Verification items for the finished model (mm, model axes). Face numbers are marked on the shaded views. A direction names the side the tool comes from. Round coordinates to 2 decimals unless told otherwise and drop trailing zeros. Write each loop counter-clockwise with the first axis right and the second up, starting at its lowest first coordinate (ties: lowest second). Pieces come first, ordered by that corner, then holes. Notation, with made-up numbers: (71.5, -23.75) - (82.5, -23.75) arc R26 cw to (82.5, -0.75) - close; hole circle Ø1 at (45.5, 78.25). An arc over 180 degrees is marked (long way). Write each question's results on one line, items separated by ' | '.
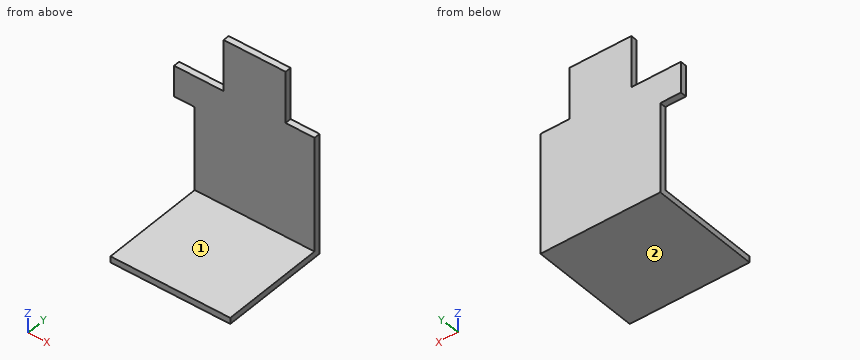
```python
from build123d import *

# Parameters (mm, degrees)
BOX015001038_W     = 58
BOX015001038_H     = 53.5
BOX015001038_DEPTH = 3
BOX015001039_W     = 10
BOX015001039_H     = 3
BOX015001039_DEPTH = 15
BOX015001041_W     = 14
BOX015001041_H     = 10
BOX015001041_DEPTH = 25
BOX015001040_W     = 14
BOX015001040_H     = 10
BOX015001040_DEPTH = 25
BOX015001037_W     = 58
BOX015001037_H     = 3
BOX015001037_DEPTH = 80.5


with BuildPart() as cube034:
    # Box015001038 → Box015001038 (new body)
    with BuildSketch(Plane(origin=(0, -50.5, -3), x_dir=(1, 0, 0), z_dir=(0, 0, 1))):
        with Locations((29, 26.75)):
            Rectangle(BOX015001038_W, BOX015001038_H)
    extrude(amount=BOX015001038_DEPTH)


with BuildPart() as cube035:
    # Box015001039 → Box015001039 (new body)
    with BuildSketch(Plane(origin=(-10, 0, 40.5), x_dir=(1, 0, 0), z_dir=(0, 0, 1))):
        with Locations((5, 1.5)):
            Rectangle(BOX015001039_W, BOX015001039_H)
    extrude(amount=BOX015001039_DEPTH)


with BuildPart() as cube037:
    # Box015001041 → Box015001041 (new body)
    with BuildSketch(Plane(origin=(44, 0, 55.5), x_dir=(1, 0, 0), z_dir=(0, 0, 1))):
        with Locations((7, 5)):
            Rectangle(BOX015001041_W, BOX015001041_H)
    extrude(amount=BOX015001041_DEPTH)


with BuildPart() as cube036:
    # Box015001040 → Box015001040 (new body)
    with BuildSketch(Plane.XY.offset(55.5)):
        with Locations((7, 5)):
            Rectangle(BOX015001040_W, BOX015001040_H)
    extrude(amount=BOX015001040_DEPTH)


with BuildPart() as fusion001019007:
    # Box015001037 → Box015001037 (new body)
    with BuildSketch(Plane.XY):
        with Locations((29, 1.5)):
            Rectangle(BOX015001037_W, BOX015001037_H)
    extrude(amount=BOX015001037_DEPTH)

    # Cut003047: cut Cube036
    add(cube036.part, mode=Mode.SUBTRACT)

    # Cut003048: cut Cube037
    add(cube037.part, mode=Mode.SUBTRACT)

    # Fusion001019006: union Cube035
    add(cube035.part)

    # Fusion001019007: union Cube034
    add(cube034.part)


solid = fusion001019007.part
```
(1) Section check B-B (z = 9). Record the cut outline in (x, y), plus the area to 3 significant figures.
Answer:
outline: (0, 0) - (58, 0) - (58, 3) - (0, 3) - close | area: 174 mm2
(2) Section check C-C (y = -38). Record the cut outline in (x, z).
Answer:
outline: (0, -3) - (58, -3) - (58, 0) - (0, 0) - close
(3) Section check A-A (x = 2.5). Record the cut outline in (y, z), plus the area to 3 significant figures.
Answer:
outline: (-50.5, -3) - (3, -3) - (3, 55.5) - (0, 55.5) - (0, 0) - (-50.5, 0) - close | area: 327 mm2
(4) Section check D-D (x = 25.5). Record the cut outline in (y, z), plus the area to 3 significant figures.
Answer:
outline: (-50.5, -3) - (3, -3) - (3, 80.5) - (0, 80.5) - (0, 0) - (-50.5, 0) - close | area: 402 mm2
(5) Set-up check for the marked faces 1 and 2: record each of +Z, -Z, +X, -X, +Y, -Y from which the full face is reachable in a straight line by a thin tool's end or side.
Answer:
face 1: +Z, +X, -X, -Y | face 2: -Z, +X, -X, +Y, -Y
(6) Thickness scan on L1, parallel to Y at x = 34, z = 61; L2, parallel to Z at x = 19.5, y = -26.5. Record the ranges inside material, lowest first.
Answer:
L1: 0 to 3 | L2: -3 to 0
(7) Go/stop test with flat-tipped pins: pin 1 Ø10 at (x, y) = (1.5, -13) entering from +Z; pin 2 Ø1.5 at (x, y) = (-4.5, 1.5) entering from -Z; pin 3 Ø10 at (y, z) = (-3, 62.5) entering from -X. Record where each tip stops, or that it passes through.
Answer:
pin 1: z = 0 | pin 2: z = 40.5 | pin 3: x = 14
